Geometry check sheet. Reference: the model listing, model coordinates, mm. Face numbers are marked on the shaded views. A direction names the side the tool comes from. Round coordinates to 2 decimals unless told otherwise and drop trailing zeros. Loops run counter-clockwise (first coordinate to the right, second up) from the corner with the lowest first, then second, coordinate; pieces in that order, holes last. Notation, with made-up numbers: (39, 20) - (83, 20) arc R9 ccw to (83, 33) - close; hole circle Ø3 at (35.25, 46.25). An arc over 180 degrees is marked (long way). Answer as CSV lines item,"result". Start each with the question number.
1) Cross-section at A-A on z = 0. Record the boundary of the cut face in (x, y), and give its area (3 significant figures).
2) Draft check along Z on the marked faces 6, 7 and 8. Enter one of: released by +Z, released by -Z, zero draft, split by the parting line, or undercut.
3) Access from +Z, -Z, +X, -X, +Y, -Y to the whole of each face (thin tool, end or side, straight path). Record for the marked faces 1, 2, 3, 4 and 5.
4) Cross-section at B-B on y = 3.65. Record the boundary of the cut face in (x, z), and give its area (3 significant figures).
5) Depth check by flat-ended pin: P1, Ø0.7, axis at x = 24, y = 3.5, coming from the -Z side; P2, Ø0.8, axis at x = 1, y = 5.5, coming from the -Z side; P3, Ø8.5, axis at x = -7.5, z = -19.5, coming from the -Y side. Enter the tip coordinate at first touch or a pass-through.
6) Cross-section at D-D on y = 1. Record the boundary of the cut face in (x, z).
7) Thickness scan on line 1 along X through (y, z) = (0.5, 0); line 2 along Z through (x, y) = (0, 5.45); line 3 along X through (y, z) = (2.9, -1.5). Record the ranges inside material, lowest first.
from build123d import *

# Parameters (mm, degrees)
BOSS_EXTRUDE1_DEPTH = 6
CUT_EXTRUDE1_DEPTH  = 10
CUT_EXTRUDE2_DEPTH  = 4
SKETCH4_W           = 21
SKETCH4_H           = 13
CUT_EXTRUDE3_DEPTH  = 1
SKETCH5_R           = 1.4
CUT_EXTRUDE4_DEPTH  = 10
CUT_EXTRUDE8_START  = -22.627416998
CUT_EXTRUDE8_DEPTH  = 45.254833996
SKETCH8_W           = 50.670468249
SKETCH8_H           = 10.499687698
SKETCH8_W_2         = 48.947034964
SKETCH8_H_2         = 10.380689976
CUT_EXTRUDE9_DEPTH  = 3


# Read off the part's stored shape, not the designer's step: Cut-Extrude8
with BuildPart() as part:
    # Sketch1 → Boss-Extrude1 (new body)
    with BuildSketch(Plane(origin=(0, 0, 0), x_dir=(1, 0, 0), z_dir=(0, 1, 0))):
        with BuildLine():
            Line((22.627416998, 8), (25, 8))
            Line((25, 8), (25, -8))
            Line((25, -8), (22.627416998, -8))
            ThreePointArc((22.627416998, -8), (0, -24), (-22.627416998, -8))
            Line((-22.627416998, -8), (-25, -8))
            Line((-25, -8), (-25, 8))
            Line((-25, 8), (-22.627416998, 8))
            ThreePointArc((-22.627416998, 8), (0, 24), (22.627416998, 8))
        make_face()
    extrude(amount=BOSS_EXTRUDE1_DEPTH)

    # Sketch2 → Cut-Extrude1 (cut)
    with BuildSketch(Plane(origin=(0, 6, 0), x_dir=(1, 0, 0), z_dir=(0, 1, 0))):
        with BuildLine():
            Line((-5.05, -4.25), (8.05, -4.25))
            Line((8.05, -4.25), (8.05, 4.25))
            Line((8.05, 4.25), (-5.05, 4.25))
            ThreePointArc((-5.05, 4.25), (-7.171320344, 3.371320344), (-8.05, 1.25))
            Line((-8.05, 1.25), (-8.05, -1.25))
            ThreePointArc((-8.05, -1.25), (-7.171320344, -3.371320344), (-5.05, -4.25))
        make_face()
    extrude(amount=-CUT_EXTRUDE1_DEPTH, mode=Mode.SUBTRACT)

    # Sketch3 → Cut-Extrude2 (cut)
    with BuildSketch(Plane(origin=(0, 6, 0), x_dir=(1, 0, 0), z_dir=(0, 1, 0))):
        with BuildLine():
            Line((-12.5, -5), (12.5, -5))
            ThreePointArc((12.5, -5), (13.914213562, -4.414213562), (14.5, -3))
            Line((14.5, -3), (14.5, 3))
            ThreePointArc((14.5, 3), (13.914213562, 4.414213562), (12.5, 5))
            Line((12.5, 5), (-12.5, 5))
            ThreePointArc((-12.5, 5), (-13.914213562, 4.414213562), (-14.5, 3))
            Line((-14.5, 3), (-14.5, -3))
            ThreePointArc((-14.5, -3), (-13.914213562, -4.414213562), (-12.5, -5))
        make_face()
    extrude(amount=-CUT_EXTRUDE2_DEPTH, mode=Mode.SUBTRACT)

    # Sketch4 → Cut-Extrude3 (cut)
    with BuildSketch(Plane(origin=(0, 6, 0), x_dir=(1, 0, 0), z_dir=(0, 1, 0))):
        Rectangle(SKETCH4_W, SKETCH4_H)
    extrude(amount=-CUT_EXTRUDE3_DEPTH, mode=Mode.SUBTRACT)

    # Sketch5 → Cut-Extrude4 (cut)
    with BuildSketch(Plane(origin=(0, 2, 0), x_dir=(1, 0, 0), z_dir=(0, 1, 0))):
        with Locations(Location((-10.25, 0, 0), (0, 0, 270))):
            Circle(SKETCH5_R)
        with Locations(Location((10.25, 0, 0), (0, 0, 270))):
            Circle(SKETCH5_R)
    extrude(amount=-CUT_EXTRUDE4_DEPTH, mode=Mode.SUBTRACT)

    # Cut-Extrude8 outline → Cut-Extrude8 (cut)
    with BuildSketch(Plane.YZ.offset(CUT_EXTRUDE8_START)):
        Polygon((0, -24.445099732), (0.162003054, -24), (2.992763401, -16.222549867), (0, -8), align=None)
        Polygon((0, 23.933160472), (0, 8), (2.899598075, 15.966580236), align=None)
    extrude(amount=CUT_EXTRUDE8_DEPTH, mode=Mode.SUBTRACT)

    # Sketch8 → Cut-Extrude9 (cut)
    with BuildSketch(Plane.XZ):
        with Locations((1.133817479, 21.216424085)):
            Rectangle(SKETCH8_W, SKETCH8_H)
        with Locations((0.272100837, -21.412894855)):
            Rectangle(SKETCH8_W_2, SKETCH8_H_2)
    extrude(amount=-CUT_EXTRUDE9_DEPTH, mode=Mode.SUBTRACT)


solid = part.part
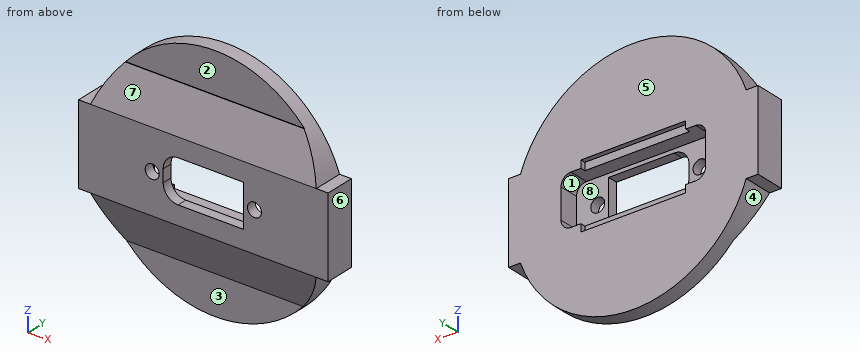
Answer block:
1,outline,"(-25, 0) - (-11.65, 0) - (-11.65, 2) - (-14.5, 2) - (-14.5, 6) - (-25, 6) - close; (-8.85, 0) - (-8.05, 0) - (-8.05, 2) - (-8.85, 2) - close; (8.05, 0) - (8.85, 0) - (8.85, 2) - (8.05, 2) - close; (11.65, 0) - (25, 0) - (25, 6) - (14.5, 6) - (14.5, 2) - (11.65, 2) - close"
1,area,"141 mm^2"
2,face 6,"zero draft"
2,face 7,"released by +Z"
2,face 8,"undercut"
3,face 1,"+Y"
3,face 2,"+Z, +X, -X, -Y"
3,face 3,"-Z, +X, -X, -Y"
3,face 4,"-Z, +Y, -Y"
3,face 5,"+Z, -Z, +X, -X, +Y"
4,outline,"(-25, -8) - (-22.63, -8) arc R24 ccw to (22.63, -8) - (25, -8) - (25, 8) - (22.63, 8) arc R24 ccw to (-22.63, 8) - (-25, 8) - close; hole (-14.5, -3) arc R2 ccw to (-12.5, -5) - (12.5, -5) arc R2 ccw to (14.5, -3) - (14.5, 3) arc R2 ccw to (12.5, 5) - (-12.5, 5) arc R2 ccw to (-14.5, 3) - close"
4,area,"1,570 mm^2"
5,P1,"stops at z = -8"
5,P2,"stops at z = -23.99"
5,P3,"stops at y = 2.64"
6,outline,"(-25, -8) - (-22.63, -8) arc R24 ccw to (-21.46, -10.75) - (21.46, -10.75) arc R24 ccw to (22.63, -8) - (25, -8) - (25, 8) - (22.63, 8) arc R24 ccw to (21.46, 10.75) - (-21.46, 10.75) arc R24 ccw to (-22.63, 8) - (-25, 8) - close; hole circle Ø2.8 at (-10.25, 0); hole (-8.05, -1.25) arc R3 ccw to (-5.05, -4.25) - (8.05, -4.25) - (8.05, 4.25) - (-5.05, 4.25) arc R3 ccw to (-8.05, 1.25) - close; hole circle Ø2.8 at (10.25, 0)"
7,line 1,"x = -25 to -11.65, -8.85 to -8.05, 8.05 to 8.85, 11.65 to 25"
7,line 2,"z = -24 to -6.5, 6.5 to 24"
7,line 3,"x = -25 to -14.5, 14.5 to 25"
